Source: CAD feature listing. Evaluate the final solid. Frame: model axes, mm. Face numbers are marked on the shaded views. A direction names the side the tool comes from. Round coordinates to 2 decimals unless told otherwise and drop trailing zeros. Loops run counter-clockwise (first coordinate to the right, second up) from the corner with the lowest first, then second, coordinate; pieces in that order, holes last.
(1) Material intervals for probe 1 along Z at (x, y) = (-6.5, -20); probe 2 along Y at (x, z) = (-4.5, 11); probe 3 along X at (y, z) = (-74.5, 8.75), sorted ascending.
(2) Section A-A, the plane x = -10.5. Return the cut outline in (y, z).
(3) Mould query, pull axis Y, two halves, no side actions, for the marked faces 3, 4, 5 and 6. Classes: pulls with the +Y half, pulls with the -Y half, needs draft (parallel to the pull), parting line crosses it, or undercut.
(4) First-contact query: pin 1 Ø2 at (x, z) = (-15.5, 17) entering from -Y; pin 2 Ø2 at (x, z) = (-17, 16.5) entering from +Y; pin 3 Ø6.5 at (y, z) = (-6.5, 7.5) entering from -X. Flat tips, straight axial feed; report the tip coordinate or a pass-through.
(5) Section B-B, the plane z = 12.5. Return the cut outline in (x, y).
(6) Section C-C, the plane y = -53.5. Return the cut outline in (x, z).
(7) Set-up query: the marked faces 1 and 2. Return all of +Z, -Z, +X, -X, +Y, -Y with unobstructed straight access to the full face (end or side cutting, diameter ignored); none if empty.
(8) Section D-D, the plane x = 5.5. Return the cut outline in (y, z).
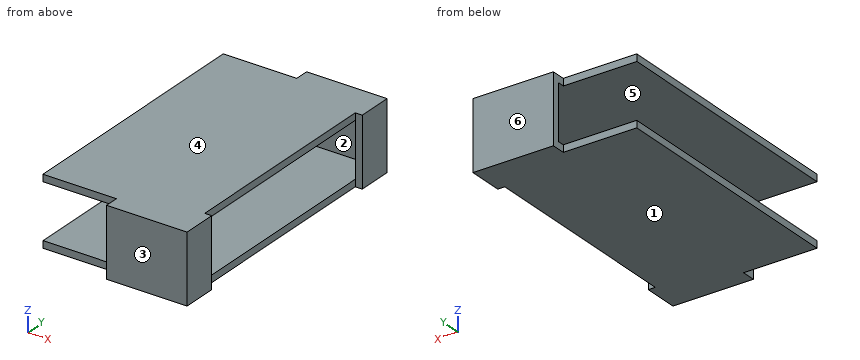
```python
from build123d import *

# Parameters (mm, degrees)
F0_W      = 18
F0_H      = 15.6
F0_H_2    = 2
F1_DEPTH  = 2
F2_W      = 18
F2_H      = 2
F3_DEPTH  = 76.9
F4_W      = 18
F4_H      = 19.6
F5_DEPTH  = 2
F6_W      = 72.9
F6_H      = 2
F7_DEPTH  = 21
F8_W      = 80.9
F8_H      = 19.6
F8_W_2    = 76.9
F8_H_2    = 15.6
F9_DEPTH  = 3
F11_DEPTH = 2
F12_W     = 2
F12_H     = 19.6
F13_DEPTH = 8
F14_W     = 2
F14_H     = 19.6
F15_DEPTH = 8


with BuildPart() as f1:
    # F0 (on Front) → F1 (new body)
    with BuildSketch(Plane.XZ):
        with Locations((2.132421, 7.8)):
            Rectangle(F0_W, F0_H)
        with Locations((2.132421, -1)):
            Rectangle(F0_W, F0_H_2)
        with Locations((2.132421, 16.6)):
            Rectangle(F0_W, F0_H_2)
    extrude(amount=F1_DEPTH)

    # F2 (on face) → F3 (join)
    with BuildSketch(Plane.XZ.offset(2)):
        with Locations((2.132421, 16.6)):
            Rectangle(F2_W, F2_H)
        with Locations((2.132421, -1)):
            Rectangle(F2_W, F2_H)
    extrude(amount=F3_DEPTH)

    # F4 (on face) → F5 (join)
    with BuildSketch(Plane.XZ.offset(78.9)):
        with Locations((2.132421, 7.8)):
            Rectangle(F4_W, F4_H)
    extrude(amount=F5_DEPTH)

    # F6 (on face) → F7 (join)
    with BuildSketch(Plane(origin=(-6.867579, 0, 0), x_dir=(0, -1, 0), z_dir=(-1, 0, 0))):
        with Locations((40.45, 16.6)):
            Rectangle(F6_W, F6_H)
        with Locations((40.45, -1)):
            Rectangle(F6_W, F6_H)
    extrude(amount=F7_DEPTH)

    # F8 (on face) → F9 (join)
    with BuildSketch(Plane.YZ.offset(11.132421)):
        with Locations((-40.45, 7.8)):
            Rectangle(F8_W, F8_H)
        with Locations((-40.45, 7.8)):
            Rectangle(F8_W_2, F8_H_2, mode=Mode.SUBTRACT)
    extrude(amount=F9_DEPTH)

    # F10 (on face) → F11 (join)
    with BuildSketch(Plane.YZ.offset(14.132421)):
        Polygon((-78.9, -2), (-78.9, 0), (-78.9, 15.6), (-78.9, 17.6), (-80.9, 17.6), (-80.9, -2), align=None)
        Polygon((-2, -2), (0, -2), (0, 17.6), (-2, 17.6), (-2, 0), align=None)
    extrude(amount=F11_DEPTH)

    # F12 (on face) → F13 (join)
    with BuildSketch(Plane(origin=(0, -78.9, 0), x_dir=(-1, 0, 0), z_dir=(0, 1, 0))):
        with Locations((-15.132421, 7.8)):
            Rectangle(F12_W, F12_H)
    extrude(amount=F13_DEPTH)

    # F14 (on face) → F15 (join)
    with BuildSketch(Plane.XZ.offset(2)):
        with Locations((15.132421, 7.8)):
            Rectangle(F14_W, F14_H)
    extrude(amount=F15_DEPTH)


solid = f1.part
```
Output values:
1. probe 1: z = -2 to 0, 15.6 to 17.6
1. probe 2: y = -80.9 to -78.9, -2 to 0
1. probe 3: x = 14.13 to 16.13
2. outline: (-76.9, -2) - (-4, -2) - (-4, 0) - (-76.9, 0) - close; (-76.9, 15.6) - (-4, 15.6) - (-4, 17.6) - (-76.9, 17.6) - close
3. face 3: pulls with the -Y half
3. face 4: needs draft
3. face 5: undercut
3. face 6: pulls with the +Y half
4. pin 1: stops at y = -76.9
4. pin 2: stops at y = -4
4. pin 3: stops at x = 14.13
5. outline: (-6.87, -80.9) - (16.13, -80.9) - (16.13, -70.9) - (14.13, -70.9) - (14.13, -78.9) - (-6.87, -78.9) - close; (-6.87, -2) - (14.13, -2) - (14.13, -10) - (16.13, -10) - (16.13, 0) - (-6.87, 0) - close
6. outline: (-27.87, -2) - (14.13, -2) - (14.13, 0) - (-27.87, 0) - close; (-27.87, 15.6) - (14.13, 15.6) - (14.13, 17.6) - (-27.87, 17.6) - close
7. face 1: -Z, +X, -X, +Y, -Y
7. face 2: -X
8. outline: (-80.9, -2) - (0, -2) - (0, 17.6) - (-80.9, 17.6) - close; hole (-78.9, 0) - (-2, 0) - (-2, 15.6) - (-78.9, 15.6) - close
